from build123d import *

# Parameters (mm, degrees)
SKETCH1_W                      = 25.4
SKETCH1_H                      = 232.968
BOSS_EXTRUDE1_DEPTH            = 6.35
M3_CLEARANCE_HOLE1_D           = 3.4
M3_CLEARANCE_HOLE1_DEPTH       = 7.493
M3_CLEARANCE_HOLE1_CSINK_D     = 3.45
M3_CLEARANCE_HOLE1_CSINK_ANGLE = 100
M3_CLEARANCE_HOLE1_TIP         = 1.021463052
M4_CLEARANCE_HOLE1_D           = 4.5
M4_CLEARANCE_HOLE1_DEPTH       = 10.1000052
M4_CLEARANCE_HOLE1_CSINK_D     = 4.55
M4_CLEARANCE_HOLE1_CSINK_ANGLE = 100
M4_CLEARANCE_HOLE1_TIP         = 1.351936393


with BuildPart() as part:
    # Sketch1 → Boss-Extrude1 (new body)
    with BuildSketch(Plane(origin=(0, 0, 0), x_dir=(0, 0, -1), z_dir=(1, 0, 0))):
        with Locations((12.7, 116.484)):
            Rectangle(SKETCH1_W, SKETCH1_H)
    extrude(amount=BOSS_EXTRUDE1_DEPTH)

    # M3 Clearance Hole1
    with Locations(Plane(origin=(6.35, 0, 0), x_dir=(0, 0, -1), z_dir=(1, 0, 0))):
        with Locations((6.7, 13.3), (18.7, 13.3)):
            CounterSinkHole(M3_CLEARANCE_HOLE1_D / 2, M3_CLEARANCE_HOLE1_CSINK_D / 2, depth=M3_CLEARANCE_HOLE1_DEPTH, counter_sink_angle=M3_CLEARANCE_HOLE1_CSINK_ANGLE)
            with Locations((0, 0, -(M3_CLEARANCE_HOLE1_DEPTH + M3_CLEARANCE_HOLE1_TIP / 2))):  # 118° drill point
                Cone(0, M3_CLEARANCE_HOLE1_D / 2, M3_CLEARANCE_HOLE1_TIP, mode=Mode.SUBTRACT)

    # M4 Clearance Hole1
    with Locations(Plane(origin=(6.35, 0, 0), x_dir=(0, 0, -1), z_dir=(1, 0, 0))):
        with Locations((4.7, 198.968), (4.7, 168.968), (4.7, 138.968), (20.7, 138.968), (20.7, 168.968), (20.7, 198.968)):
            CounterSinkHole(M4_CLEARANCE_HOLE1_D / 2, M4_CLEARANCE_HOLE1_CSINK_D / 2, depth=M4_CLEARANCE_HOLE1_DEPTH, counter_sink_angle=M4_CLEARANCE_HOLE1_CSINK_ANGLE)
            with Locations((0, 0, -(M4_CLEARANCE_HOLE1_DEPTH + M4_CLEARANCE_HOLE1_TIP / 2))):  # 118° drill point
                Cone(0, M4_CLEARANCE_HOLE1_D / 2, M4_CLEARANCE_HOLE1_TIP, mode=Mode.SUBTRACT)


solid = part.part
For this review, take the finished solid that the model builds, in its own axes (mm). Round coordinates to 2 decimals unless told otherwise and drop trailing zeros. Use a Markdown table: item, result.
Q1. Clearance check with a flat-ended pin moving along its axis: pin 1 (2.5 mm diameter, centred on y = 168.968, z = -20.7, fed in from -X). State where the tip first meets the part, or that it passes through.
Derived:
| item | result |
|---|---|
| pin 1 | passes through |
Q2. We need section A-A (x = 2). State how many separate pieces and enclosed holes the cut face has, plus the area to 3 significant figures.
Derived:
| item | result |
|---|---|
| separate pieces | 1 |
| enclosed holes | 8 |
| area | 5,800 mm2 |
Q3. The part is to be moulded in two halves that separate along Y. For faces 1 (the flat face through (3, 115, 0)), 2 (the cylindrical face through (3.12, 197.599, -22.486)), 3 (the flat face through (3, 0, -13)), say which applies: pulls with the +Y half, pulls with the -Y half, needs draft (parallel to the pull), parting line crosses it, or undercut.
Derived:
| item | result |
|---|---|
| face 1 | needs draft |
| face 2 | undercut |
| face 3 | pulls with the -Y half |
Q4. Wall thickness on line 1 along Y through (x, z) = (4.25, -4.7); line 2 along Z through (x, y) = (1.5, 13.3); line 3 along Y through (x, z) = (3.5, -18.7): over which ranges is each line inside the solid? List them lowest first.
Derived:
| item | result |
|---|---|
| line 1 | y = 0 to 136.72, 141.22 to 166.72, 171.22 to 196.72, 201.22 to 232.97 |
| line 2 | z = -25.4 to -20.4, -17 to -8.4, -5 to 0 |
| line 3 | y = 0 to 11.6, 15 to 137.94, 140 to 167.94, 170 to 197.94, 200 to 232.97 |
